Geometry check sheet. Reference: the model listing, model coordinates, mm. Coordinates: 2 decimals unless noted, no trailing zeros. Write each loop counter-clockwise with the first axis right and the second up, starting at its lowest first coordinate (ties: lowest second). Pieces come first, ordered by that corner, then holes. Notation, with made-up numbers: (34.25, -26.5) - (41.25, -26.5) arc R23 ccw to (41.25, 7.5) - close; hole circle Ø3 at (24, -39.5). An arc over 180 degrees is marked (long way). Answer as a JSON object with one key per item and string values. Group by question number.
from build123d import *

# Parameters (mm, degrees)
CROQUIS1_R              = 0.7
CROQUIS1_R_2            = 1.25
SALIENTE_EXTRUIR1_DEPTH = 1.5


with BuildPart() as part:
    # Croquis1 → Saliente-Extruir1 (new body)
    with BuildSketch(Plane.XY):
        with BuildLine():
            Line((29.5, -15), (-29.5, -15))
            ThreePointArc((-29.5, -15), (-31.621320344, -14.121320344), (-32.5, -12))
            Line((-32.5, -12), (-32.5, 12))
            ThreePointArc((-32.5, 12), (-31.621320344, 14.121320344), (-29.5, 15))
            Line((-29.5, 15), (29.5, 15))
            ThreePointArc((29.5, 15), (31.621320344, 14.121320344), (32.5, 12))
            Line((32.5, 12), (32.5, -12))
            ThreePointArc((32.5, -12), (31.621320344, -14.121320344), (29.5, -15))
        make_face()
        with Locations((-24.13, -10.73)):
            Circle(CROQUIS1_R, mode=Mode.SUBTRACT)
        with Locations((-24.13, -13.27)):
            Circle(CROQUIS1_R, mode=Mode.SUBTRACT)
        with Locations((-21.59, -10.73)):
            Circle(CROQUIS1_R, mode=Mode.SUBTRACT)
        with Locations((-21.59, -13.27)):
            Circle(CROQUIS1_R, mode=Mode.SUBTRACT)
        with Locations((-19.05, -10.73)):
            Circle(CROQUIS1_R, mode=Mode.SUBTRACT)
        with Locations((-19.05, -13.27)):
            Circle(CROQUIS1_R, mode=Mode.SUBTRACT)
        with Locations((-16.51, -10.73)):
            Circle(CROQUIS1_R, mode=Mode.SUBTRACT)
        with Locations((-16.51, -13.27)):
            Circle(CROQUIS1_R, mode=Mode.SUBTRACT)
        with Locations((-13.97, -10.73)):
            Circle(CROQUIS1_R, mode=Mode.SUBTRACT)
        with Locations((-13.97, -13.27)):
            Circle(CROQUIS1_R, mode=Mode.SUBTRACT)
        with Locations((-11.43, -10.73)):
            Circle(CROQUIS1_R, mode=Mode.SUBTRACT)
        with Locations((-11.43, -13.27)):
            Circle(CROQUIS1_R, mode=Mode.SUBTRACT)
        with Locations((-8.89, -10.73)):
            Circle(CROQUIS1_R, mode=Mode.SUBTRACT)
        with Locations((-8.89, -13.27)):
            Circle(CROQUIS1_R, mode=Mode.SUBTRACT)
        with Locations((-6.35, -10.73)):
            Circle(CROQUIS1_R, mode=Mode.SUBTRACT)
        with Locations((-6.35, -13.27)):
            Circle(CROQUIS1_R, mode=Mode.SUBTRACT)
        with Locations((-3.81, -10.73)):
            Circle(CROQUIS1_R, mode=Mode.SUBTRACT)
        with Locations((-3.81, -13.27)):
            Circle(CROQUIS1_R, mode=Mode.SUBTRACT)
        with Locations((-1.27, -10.73)):
            Circle(CROQUIS1_R, mode=Mode.SUBTRACT)
        with Locations((-1.27, -13.27)):
            Circle(CROQUIS1_R, mode=Mode.SUBTRACT)
        with Locations((1.27, -10.73)):
            Circle(CROQUIS1_R, mode=Mode.SUBTRACT)
        with Locations((1.27, -13.27)):
            Circle(CROQUIS1_R, mode=Mode.SUBTRACT)
        with Locations((3.81, -10.73)):
            Circle(CROQUIS1_R, mode=Mode.SUBTRACT)
        with Locations((3.81, -13.27)):
            Circle(CROQUIS1_R, mode=Mode.SUBTRACT)
        with Locations((6.35, -10.73)):
            Circle(CROQUIS1_R, mode=Mode.SUBTRACT)
        with Locations((6.35, -13.27)):
            Circle(CROQUIS1_R, mode=Mode.SUBTRACT)
        with Locations((8.89, -10.73)):
            Circle(CROQUIS1_R, mode=Mode.SUBTRACT)
        with Locations((8.89, -13.27)):
            Circle(CROQUIS1_R, mode=Mode.SUBTRACT)
        with Locations((11.43, -10.73)):
            Circle(CROQUIS1_R, mode=Mode.SUBTRACT)
        with Locations((11.43, -13.27)):
            Circle(CROQUIS1_R, mode=Mode.SUBTRACT)
        with Locations((13.97, -10.73)):
            Circle(CROQUIS1_R, mode=Mode.SUBTRACT)
        with Locations((13.97, -13.27)):
            Circle(CROQUIS1_R, mode=Mode.SUBTRACT)
        with Locations((16.51, -10.73)):
            Circle(CROQUIS1_R, mode=Mode.SUBTRACT)
        with Locations((16.51, -13.27)):
            Circle(CROQUIS1_R, mode=Mode.SUBTRACT)
        with Locations((19.05, -10.73)):
            Circle(CROQUIS1_R, mode=Mode.SUBTRACT)
        with Locations((19.05, -13.27)):
            Circle(CROQUIS1_R, mode=Mode.SUBTRACT)
        with Locations((21.59, -10.73)):
            Circle(CROQUIS1_R, mode=Mode.SUBTRACT)
        with Locations((21.59, -13.27)):
            Circle(CROQUIS1_R, mode=Mode.SUBTRACT)
        with Locations((24.13, -10.73)):
            Circle(CROQUIS1_R, mode=Mode.SUBTRACT)
        with Locations((24.13, -13.27)):
            Circle(CROQUIS1_R, mode=Mode.SUBTRACT)
        with Locations((-29, 11.5)):
            Circle(CROQUIS1_R_2, mode=Mode.SUBTRACT)
        with Locations(Location((29, 11.5, 0), (0, 0, 180))):
            Circle(CROQUIS1_R_2, mode=Mode.SUBTRACT)
        with Locations((29, -11.5)):
            Circle(CROQUIS1_R_2, mode=Mode.SUBTRACT)
        with Locations(Location((-29, -11.5, 0), (0, 0, 180))):
            Circle(CROQUIS1_R_2, mode=Mode.SUBTRACT)
    extrude(amount=SALIENTE_EXTRUIR1_DEPTH)


solid = part.part
(1) Material ranges on L1, parallel to Y at x = -24.13, z = 1.15; L2, parallel to Y at x = -24.5, z = 0.8, recorded low to high. Write a range as [from, to].
(2) Section check A-A (x = -24.13). Record the cut outline in (y, z).
(3) Section check B-B (z = 0.65). Count the separate pieces of the cut face and the enclosed holes in it, and give its area (3 significant figures).
(4) Gauge pin test, flat end, axial feed: pin 1 (1.3 mm diameter, centred on x = -8.89, y = -13.27, fed in from +Z). Record the tip position at first contact, or that the pin passes through.
(5) Draft check along Y on faces 1 (the face through (-19.141, -12.576, 0.74)), 2 (the face through (32.5, 0, 1)), 3 (the face through (0, -15, 1)). Enter one of: +Y half, -Y half, draft (parallel to the pull), parting line (faces both ways), or undercut.
Conclusion:
{
 "1": {"L1": "y = [-15, -13.97], [-12.57, -11.43], [-10.03, 15]", "L2": "y = [-15, -13.86], [-12.68, -11.32], [-10.14, 15]"},
 "2": {"outline": "(-15, 0) - (-13.97, 0) - (-13.97, 1.5) - (-15, 1.5) - close; (-12.57, 0) - (-11.43, 0) - (-11.43, 1.5) - (-12.57, 1.5) - close; (-10.03, 0) - (15, 0) - (15, 1.5) - (-10.03, 1.5) - close"},
 "3": {"separate pieces": "1", "enclosed holes": "44", "area": "1,860 mm^2"},
 "4": {"pin 1": "passes through"},
 "5": {"face 1": "undercut", "face 2": "draft", "face 3": "-Y half"}
}
